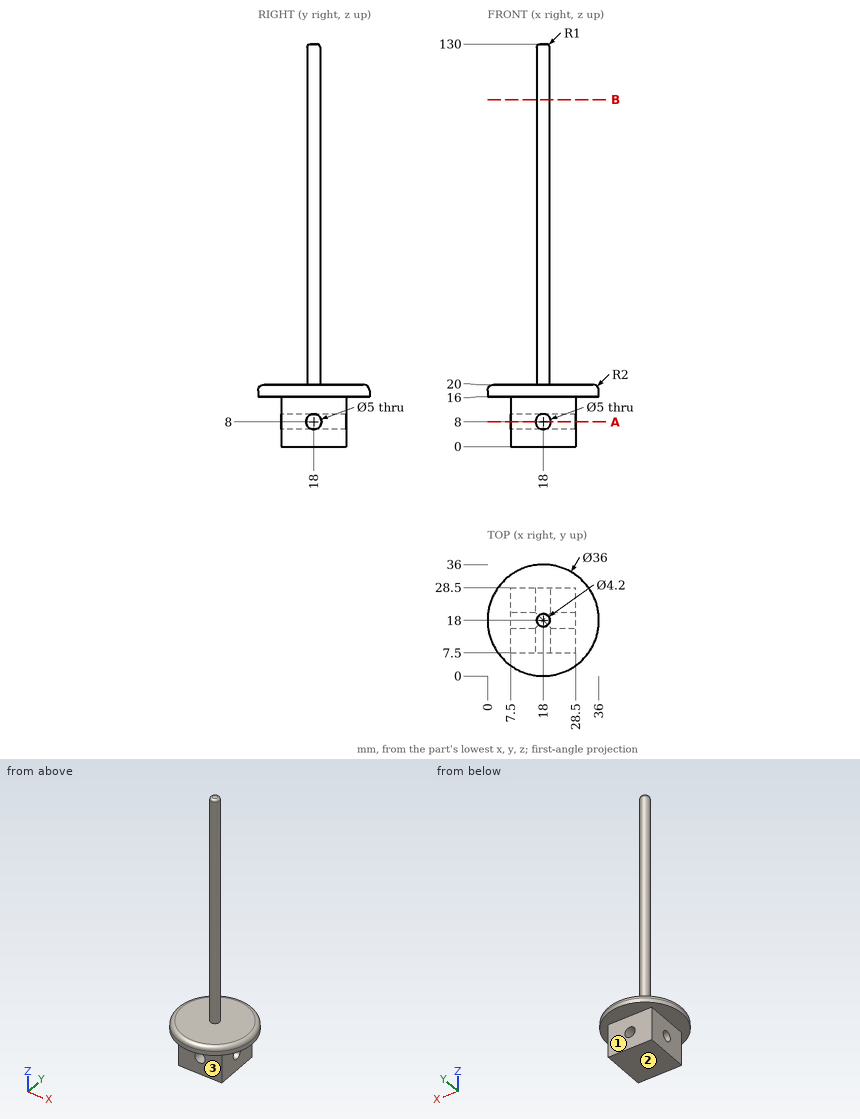
Geometry: see drawing. Coordinates: mm, zero at the bounding-box minimum. A direction names the side the tool comes from. Coordinates: 2 decimals unless noted, no trailing zeros. Loops run counter-clockwise (first coordinate to the right, second up) from the corner with the lowest first, then second, coordinate; pieces in that order, holes last. Notation, with made-up numbers: (-37, -25) -> (-26, -25) arc R37 ccw to (-26, 13) -> close; hole circle Ø5 at (-19.5, 89.25). An arc over 180 degrees is marked (long way). Write item = value, one per line. Start each with the question number.
Item 1: First-contact query: P1, Ø1, axis at x = 6, y = 19.5, coming from the -Z side; P2, Ø16, axis at x = 13.5, y = 24, coming from the +Z side; P3, Ø5, axis at y = 16, z = 11.5, coming from the -X side; P4, Ø17.5, axis at x = 21.5, z = 11.5, coming from the +Y side. Flat tips, straight axial feed; report the tip coordinate or a pass-through.
Item 2: Reachability of the marked faces 1, 2 and 3 from +Z, -Z, +X, -X, +Y, -Y: full face, straight path, thin tool, end or side. Return the list, or none.
Item 3: Cut plane B-B, the plane z = 112. Return loops of the section in (x, y).
Item 4: Cut plane A-A, the plane z = 8. Return loops of the section in (x, y), plus the area to 3 significant figures.
Item 5: Material intervals for line 1 (Z direction, x = 18, y = 15.5); line 2 (X direction, y = 14, z = 8); line 3 (X direction, y = 10, z = 12.5), sorted ascending.
Ans:
q1.P1 = 16
q1.P2 = 130
q1.P3 = 7.5
q1.P4 = 36
q2.face_1 = -Z, +X, -X, +Y
q2.face_2 = -Z, +X, -X, +Y, -Y
q2.face_3 = -Z, +X, -X, -Y
q3.outline = circle Ø4.2 at (18, 18)
q4.outline = (7.5, 7.5) -> (15.5, 7.5) -> (15.5, 15.5) -> (7.5, 15.5) -> close; (7.5, 20.5) -> (15.5, 20.5) -> (15.5, 28.5) -> (7.5, 28.5) -> close; (20.5, 7.5) -> (28.5, 7.5) -> (28.5, 15.5) -> (20.5, 15.5) -> close; (20.5, 20.5) -> (28.5, 20.5) -> (28.5, 28.5) -> (20.5, 28.5) -> close
q4.area = 256 mm²
q5.line_1 = 0 to 5.5, 10.5 to 20
q5.line_2 = 7.5 to 15.5, 20.5 to 28.5
q5.line_3 = 7.5 to 28.5
